Autodesk Inventor part; units mm, degrees
ref_plane "YZ Plane" through (0, 0, 0) normal (1, 0, 0) x (0, 1, 0)
ref_plane "XZ Plane" through (0, 0, 0) normal (0, 1, 0) x (-1, 0, 0)
ref_plane "XY Plane" through (0, 0, 0) normal (0, 0, 1) x (1, 0, 0)
sketch "Sketch1" plane through (0, 0, 0) normal (0, 1, 0) x (-1, 0, 0)
  circle A0 centre (0, 0) radius 1
  dimension "d0" = 2
extrude "Extrusion1" add sketch "Sketch1" along normal blind 20
sketch "Sketch2" plane through (0, 20, 0) normal (0, 1, 0) x (1, 0, 0)
  circle A0 centre (0, 0) radius 2
  dimension "d3" = 4
extrude "Extrusion2" add sketch "Sketch2" along normal blind 2
sketch "Sketch3" plane through (0, 22, 0) normal (0, 1, 0) x (1, 0, 0)
  circle A0 centre (0, 0) radius 1
  line L0 (0, 1) -> (0.866, 0.5)
  line L1 (0.866, 0.5) -> (0.866, -0.5)
  line L2 (0.866, -0.5) -> (0, -1)
  line L3 (0, -1) -> (-0.866, -0.5)
  line L4 (-0.866, -0.5) -> (-0.866, 0.5)
  line L5 (-0.866, 0.5) -> (0, 1)
extrude "Extrusion3" cut sketch "Sketch3" against normal blind 1 contours L1 L2 L3 L4 L5 L0
properties part number "M2_bolt"
CAD build for the part. Positions are in the model's coordinates, mm. A direction names the side the tool comes from. Give positions to 0.01 mm unless a question says otherwise; leave off trailing zeros. Order: outer loops, then holes, each group sorted by start corner. A loop starts at its lowest first (then second) coordinate and runs counter-clockwise, first axis right, second up. Notation, with made-up numbers: M -40,25 L -7,25 A31 ccw -7,54 Z; hole C -3,85.5 d2. An arc over 180 degrees is marked long. Put each result on its own line as item: value. Start each with the question number.
(1) Saw through at B-B, the plane x = -0.2. Write the cut outline in (y, z).
(2) Flat gauge pins, fed straight in: pin 1 Ø1.5 at (y, z) = (18, 0.5) entering from +X; pin 2 Ø0.5 at (x, z) = (0.5, 0) entering from +Y. Where does each tip first touch, or does it go through?
(3) Drill centre lines: line 1 along Y through (x, z) = (-0.05, -0.9); line 2 along Y through (x, z) = (-0.3, -1.7); line 3 along X through (y, z) = (5.75, -0.05). Where is each one in solid material? Low to high.
(4) Mould opens along X. For faces 1 (the flat face through (0, 0, 0)), 2 (the flat face through (0.43, 21.51, -0.75)), 3 (the cylindrical face through (0, 10, 1)) say: +X half, -X half, draft (parallel to the pull), parting line (faces both ways), or undercut.
(5) Saw through at C-C, the plane y = 11. Write the cut outline in (x, z).
(6) Saw through at A-A, the plane z = 0. Write the cut outline in (x, y).
(7) Which spindle directions (+Z, -Z, +X, -X, +Y, -Y) get a long thin tool onto all of the face, cutting with end or side? Do faces 4 (the flat face through (-0.5, 22, 0.9)), 5 (the flat face through (1, 20, 1)), 6 (the flat face through (-0.439, 21.507, -0.746)). Say none if no direction does.
(8) Saw through at D-D, the plane x = -1.25. Write the cut outline in (y, z), then the cut area to 4 significant figures.
Check result:
1. outline: M 0,-0.98 L 20,-0.98 L 20,-1.99 L 22,-1.99 L 22,-0.88 L 21,-0.88 L 21,0.88 L 22,0.88 L 22,1.99 L 20,1.99 L 20,0.98 L 0,0.98 Z
2. pin 1: stops at x = 1
2. pin 2: stops at y = 21
3. line 1: y = 0 to 21
3. line 2: y = 20 to 22
3. line 3: x = -1 to 1
4. face 1: draft
4. face 2: undercut
4. face 3: parting line
5. outline: C 0,0 d2
6. outline: M -2,20 L -1,20 L -1,0 L 1,0 L 1,20 L 2,20 L 2,22 L 0.87,22 L 0.87,21 L -0.87,21 L -0.87,22 L -2,22 Z
7. face 4: +Z, -Z, +X, -X, +Y
7. face 5: -Y
7. face 6: +Y
8. outline: M 20,-1.56 L 22,-1.56 L 22,1.56 L 20,1.56 Z
8. area: 6.245 mm2
